from build123d import *

# Parameters (mm, degrees)
SKETCH1_W               = 4.7625
SKETCH1_H               = 3.175
CUT_EXTRUDE1_DEPTH      = 17.497783942
CUT_EXTRUDE1_DEPTH_BACK = 17.497783942
SKETCH2_R               = 3.81


with BuildPart() as part:
    # Sketch1 → Revolve1 (revolve)
    with BuildSketch(Plane.XY, mode=Mode.PRIVATE) as revolve1_sk:
        Polygon((-4.7625, 0), (0, 0), (0, 9.525), (-4.7625, 9.525), (-4.7625, 3.175), align=None)
        with Locations((7.14375, 1.5875)):
            Rectangle(SKETCH1_W, SKETCH1_H)
        with Locations((-7.14375, 1.5875)):
            Rectangle(SKETCH1_W, SKETCH1_H)
        Polygon((0, 9.525), (0, 0), (4.7625, 0), (4.7625, 3.175), (4.7625, 9.525), align=None)
    revolve(revolve1_sk.sketch.rotate(Axis((-4.7625, 0, 0), (1, 0, 0)), 90), axis=Axis((-4.7625, 0, 0), (1, 0, 0)))

    # Sketch2 → Cut-Extrude1 (cut, two sides: drawn at the far end of the back side and taken through both)
    with BuildSketch(Plane(origin=(0, 0, 0), x_dir=(1, 0, 0), z_dir=(0, 1, 0)).offset(-CUT_EXTRUDE1_DEPTH_BACK)):
        with Locations(Location((0, 0, 0), (0, 0, 270))):
            Circle(SKETCH2_R)
    extrude(amount=CUT_EXTRUDE1_DEPTH + CUT_EXTRUDE1_DEPTH_BACK, mode=Mode.SUBTRACT)


solid = part.part
CAD build for the part. Positions are in the model's coordinates, mm. A direction names the side the tool comes from. Round coordinates to 2 decimals unless told otherwise and drop trailing zeros. Write each loop counter-clockwise with the first axis right and the second up, starting at its lowest first coordinate (ties: lowest second). Pieces come first, ordered by that corner, then holes.
(1) Slice it at D-D, the plane x = 2.5. Write the cut outline in (y, z) (3 decimals), and give its area (3 significant figures).
(2) Mould opens along X. For faces 4 (the face through (9.525, 0, 0)), 5 (the face through (7.18, 1.93, -2.52)), 6 (the face through (3.778, -0.133, -0.496)), 7 (the face through (-4.762, 0, 4)) say: pulls with the +X half, pulls with the -X half, needs draft (parallel to the pull), parting line crosses it, or undercut.
(3) Slice it at C-C, the plane z = -2. Write the cut outline in (x, y) (1 decimal), and give its area (3 significant figures).
(4) Slice it at A-A, the plane z = 0. Write the cut outline in (x, y) (1 decimal).
(5) 3-axis set-ups, long thin cutter, end or side, ignore diameter. For faces 1 (the face through (4.762, 0, -4)), 2 (the face through (-9.525, 0, 0)), 3 (the face through (-7.11, 1.93, -2.52)): which of +Z, -Z, +X, -X, +Y, -Y reach the whole face in a straight line?
(6) Slice it at B-B, the plane y = 2.5. Write the cut outline in (x, z) (1 decimal).
(7) Probe line 1 along X through (y, z) = (-3, 0) (3 decimals); line 2 along Z through (x, y) = (0, 3.5); line 3 along Z through (x, y) = (-3.25, -0.75). List the from-to ranges inside material, lowest first.
(8) Drop flat-ended pins along their axis: P1, Ø1, axis at x = 3.5, y = -5, coming from the +Z side (3 decimals); P2, Ø6, axis at x = 4.5, y = -7, coming from the -Z side; P3, Ø3, axis at y = 6.5, z = 0, coming from the +X side; P4, Ø1, axis at x = 5.5, z = -4, coming from the +Y side. Give the stop position or say it passes through.
From the geometry:
1. outline: (-9.081, -2.875) arc R9.525 ccw to (9.081, -2.875) - close; (-9.081, 2.875) - (9.081, 2.875) arc R9.525 ccw to start
1. area: 177 mm2
2. face 4: pulls with the +X half
2. face 5: needs draft
2. face 6: undercut
2. face 7: pulls with the -X half
3. outline: (-9.5, -2.5) - (-4.8, -2.5) - (-4.8, -9.3) - (-3.2, -9.3) - (-3.2, 9.3) - (-4.8, 9.3) - (-4.8, 2.5) - (-9.5, 2.5) - close; (3.2, -9.3) - (4.8, -9.3) - (4.8, -2.5) - (9.5, -2.5) - (9.5, 2.5) - (4.8, 2.5) - (4.8, 9.3) - (3.2, 9.3) - close
3. area: 104 mm2
4. outline: (-9.5, -3.2) - (-4.8, -3.2) - (-4.8, -9.5) - (-3.8, -9.5) - (-3.8, 9.5) - (-4.8, 9.5) - (-4.8, 3.2) - (-9.5, 3.2) - close; (3.8, -9.5) - (4.8, -9.5) - (4.8, -3.2) - (9.5, -3.2) - (9.5, 3.2) - (4.8, 3.2) - (4.8, 9.5) - (3.8, 9.5) - close
5. face 1: +X
5. face 2: +Z, -Z, -X, +Y, -Y
5. face 3: -X
6. outline: (-9.5, -2) - (-4.8, -2) - (-4.8, -9.2) - (4.8, -9.2) - (4.8, -2) - (9.5, -2) - (9.5, 2) - (4.8, 2) - (4.8, 9.2) - (-4.8, 9.2) - (-4.8, 2) - (-9.5, 2) - close; hole circle Ø7.6 at (0, 0)
7. line 1: x = -9.525 to -3.81, 3.81 to 9.525
7. line 2: z = -8.86 to -3.81, 3.81 to 8.86
7. line 3: z = -9.5 to -1.99, 1.99 to 9.5
8. P1: stops at z = 8.395
8. P2: stops at z = -8.64
8. P3: stops at x = 4.76
8. P4: passes through
